from build123d import *

# Parameters (mm, degrees)
BASE_FLANGE1_DEPTH              = 0.5
SKETCH2_W                       = 1968.518691842
SKETCH2_H                       = 782.123286761
CUT_EXTRUDE1_DEPTH              = 10
CUT_EXTRUDE3_DEPTH              = 10
SKETCH10_R                      = 3.5
CUT_EXTRUDE4_DEPTH              = 10
CIRPATTERN1_COUNT               = 10
CIRPATTERN1_ANGLE               = 94.5
CIRPATTERN1_THE_OTHER_WAY_COUNT = 10
CIRPATTERN1_THE_OTHER_WAY_ANGLE = 94.5


# Sheet-metal steps are written as plain solids
with BuildPart() as part:
    # Sketch1 → Base-Flange1 (new body)
    with BuildSketch(Plane.XY):
        with BuildLine():
            Line((859.985464993, -5), (-859.985464993, -5))
            ThreePointArc((-859.985464993, -5), (0, -860), (859.985464993, -5))
        make_face()
    extrude(amount=-BASE_FLANGE1_DEPTH)

    # Sketch2 → Cut-Extrude1 (cut)
    with BuildSketch(Plane.XY):
        with Locations((10.387961435, 27.061643381)):
            Rectangle(SKETCH2_W, SKETCH2_H)
    extrude(amount=-CUT_EXTRUDE1_DEPTH, mode=Mode.SUBTRACT)

    # Sketch9 → Cut-Extrude3 (cut)
    with BuildSketch(Plane.XY):
        with BuildLine():
            Line((-723.60486455, -364), (723.60486455, -364))
            ThreePointArc((723.60486455, -364), (0, -810), (-723.60486455, -364))
        make_face()
    extrude(amount=-CUT_EXTRUDE3_DEPTH, mode=Mode.SUBTRACT)

    # Sketch10 → Cut-Extrude4 (cut)
    with BuildSketch(Plane(origin=(0, 0, -0.5), x_dir=(-1, 0, 0), z_dir=(0, 0, -1))):
        with Locations((0, -820)):
            Circle(SKETCH10_R)
    cut_extrude4 = extrude(amount=-CUT_EXTRUDE4_DEPTH, mode=Mode.SUBTRACT)

    # CirPattern1: Cut-Extrude4 ×10 about axis
    cirpattern1_axis = Axis((0, 0, 0), (0, 0, 1))
    for i in range(1, CIRPATTERN1_COUNT):
        add(cut_extrude4.rotate(cirpattern1_axis, i * CIRPATTERN1_ANGLE / (CIRPATTERN1_COUNT - 1)), mode=Mode.SUBTRACT)

    # CirPattern1 the other way: Cut-Extrude4 ×10 about axis
    cirpattern1_the_other_way_axis = Axis((0, 0, 0), (0, 0, -1))
    for i in range(1, CIRPATTERN1_THE_OTHER_WAY_COUNT):
        add(cut_extrude4.rotate(cirpattern1_the_other_way_axis, i * CIRPATTERN1_THE_OTHER_WAY_ANGLE / (CIRPATTERN1_THE_OTHER_WAY_COUNT - 1)), mode=Mode.SUBTRACT)


solid = part.part
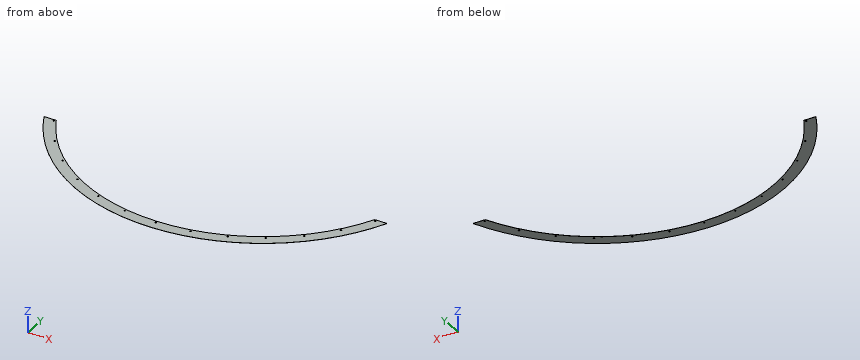
Check sheet for the modelled part. Datum: model origin and axes. Units: mm. Give positions to 0.01 mm unless a question says otherwise; leave off trailing zeros. Order: outer loops, then holes, each group sorted by start corner. A loop starts at its lowest first (then second) coordinate and runs counter-clockwise, first axis right, second up. Notation, with made-up numbers: M 61.5,43.5 L 87.5,43.5 A23 cw 87.5,70.5 Z; hole C -38,57 d10. An arc over 180 degrees is marked long. Answer as CSV lines item,"result". Start each with the question number.
Item 1: Thickness scan on line 1 (X direction, y = -444.5, z = -0.2); line 2 (X direction, y = -489.5, z = -0.3); line 3 (Y direction, x = -649, z = -0.05). Record the ranges inside material, lowest first. Write a range as [from, to].
Item 2: Cross-section at B-B on z = -0.2. State how many separate pieces and enclosed holes the cut face has, plus the area to 3 significant figures.
Item 3: Cross-section at C-C on y = -461. Enter the section's corners in (x, z), plus the area to 3 significant figures.
Item 4: Gauge pin test, flat end, axial feed: P1, Ø1.5, axis at x = -511.5, y = -631, coming from the +Z side. Record the tip position at first contact, or that the pin passes through.
Item 5: Cross-section at A-A on y = -745.5. Enter the section's corners in (x, z).
Item 6: Cross-section at D-D on x = 49. Enter the section's corners in (y, z).
Established:
1,line 1,"x = [-736.22, -677.14], [677.14, 736.22]"
1,line 2,"x = [-707.1, -645.36], [645.36, 707.1]"
1,line 3,"y = [-564.27, -502.32], [-496.05, -484.66]"
2,separate pieces,"1"
2,enclosed holes,"13"
2,area,"93,000 mm^2"
3,outline,"M -726,-0.5 L -666.02,-0.5 L -666.02,0 L -726,0 Z; M 666.02,-0.5 L 726,-0.5 L 726,0 L 666.02,0 Z"
3,area,"60.0 mm^2"
4,P1,"stops at z = 0"
5,outline,"M -428.75,-0.5 L -316.75,-0.5 L -316.75,0 L -428.75,0 Z; M 316.75,-0.5 L 428.75,-0.5 L 428.75,0 L 316.75,0 Z"
6,outline,"M -858.6,-0.5 L -808.52,-0.5 L -808.52,0 L -858.6,0 Z"
